```python
from build123d import *

# Parameters (mm, degrees)
SKETCH1_R           = 31.75
SKETCH1_R_2         = 2.05
SKETCH1_R_3         = 1.55
BOSS_EXTRUDE1_DEPTH = 40
SKETCH2_R           = 6.5
CUT_EXTRUDE1_DEPTH  = 30


with BuildPart() as part:
    # Sketch1 → Boss-Extrude1 (new body)
    with BuildSketch(Plane(origin=(0, 0, 0), x_dir=(1, 0, 0), z_dir=(0, 1, 0))):
        with Locations(Location((0, 0, 0), (0, 0, 270))):
            Circle(SKETCH1_R)
        with Locations(Location((0, 0, 0), (0, 0, 270))):
            Circle(SKETCH1_R_2, mode=Mode.SUBTRACT)
        with Locations(Location((0, 12.5, 0), (0, 0, 270))):
            Circle(SKETCH1_R_3, mode=Mode.SUBTRACT)
        with Locations(Location((12.5, 0, 0), (0, 0, 270))):
            Circle(SKETCH1_R_3, mode=Mode.SUBTRACT)
        with Locations(Location((0, -12.5, 0), (0, 0, 270))):
            Circle(SKETCH1_R_3, mode=Mode.SUBTRACT)
        with Locations(Location((-12.5, 0, 0), (0, 0, 270))):
            Circle(SKETCH1_R_3, mode=Mode.SUBTRACT)
        with Locations(Location((19.083044257, 19.083044257, 0), (0, 0, 270))):
            Circle(SKETCH1_R_3, mode=Mode.SUBTRACT)
        with Locations(Location((19.083044257, -19.083044257, 0), (0, 0, 270))):
            Circle(SKETCH1_R_3, mode=Mode.SUBTRACT)
        with Locations(Location((-19.083044257, -19.083044257, 0), (0, 0, 270))):
            Circle(SKETCH1_R_3, mode=Mode.SUBTRACT)
        with Locations(Location((-19.083044257, 19.083044257, 0), (0, 0, 270))):
            Circle(SKETCH1_R_3, mode=Mode.SUBTRACT)
    extrude(amount=BOSS_EXTRUDE1_DEPTH)

    # Sketch2 → Cut-Extrude1 (cut)
    with BuildSketch(Plane.XZ):
        with Locations(Location((0, 0, 0), (0, 0, 270))):
            Circle(SKETCH2_R)
    extrude(amount=-CUT_EXTRUDE1_DEPTH, mode=Mode.SUBTRACT)


solid = part.part
```
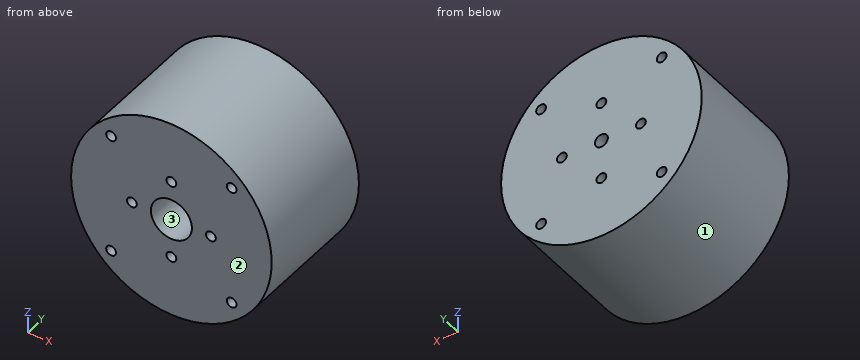
Here's how the part is built. I have some questions about the finished solid (model axes, mm). Face numbers are marked on the shaded views. Give positions to 0.01 mm unless a question says otherwise; leave off trailing zeros. Write each loop counter-clockwise with the first axis right and the second up, starting at its lowest first coordinate (ties: lowest second). Pieces come first, ordered by that corner, then holes.
(1) Imagine slicing it at C-C, the plane y = 7. Count the separate pieces of the cut face and the enclosed holes in it, and give its area (3 significant figures).
Output values:
separate pieces: 1
enclosed holes: 9
area: 2,970 mm2
(2) Imagine slicing it at D-D, the plane x = 12.5. Write out the boundary of the cut face in (y, z).
Output values:
outline: (0, -29.19) - (40, -29.19) - (40, -1.55) - (0, -1.55) - close; (0, 1.55) - (40, 1.55) - (40, 29.19) - (0, 29.19) - close
(3) If I drill on L1, parallel to X at y = 23.75, z = 0; L2, parallel to X at y = 38, z = 20.5; L3, parallel to X at y = 14, z = -12.5, over which ranges is the centre line in solid material (lowest first)?
Output values:
L1: x = -31.75 to -14.05, -10.95 to -6.5, 6.5 to 10.95, 14.05 to 31.75
L2: x = -24.24 to -19.71, -18.45 to 18.45, 19.71 to 24.24
L3: x = -29.19 to -1.55, 1.55 to 29.19
(4) Imagine slicing it at B-B, the plane z = -12.5. Write out the boundary of the cut face in (x, y).
Output values:
outline: (-29.19, 0) - (-1.55, 0) - (-1.55, 40) - (-29.19, 40) - close; (1.55, 0) - (29.19, 0) - (29.19, 40) - (1.55, 40) - close
(5) Will these pins go through, and if not, where does the flat tip stop? pin 1 (3 mm diameter, centred on x = 12.5, y = 8.5, fed in from +Z); pin 2 (5 mm diameter, centred on y = 29, z = -17, fed in from +X); pin 3 (2.5 mm diameter, centred on x = 19.08, z = -19.08, fed in from +Y); pin 4 (4 mm diameter, centred on x = -1.5, z = -2.5, fed in from -Y).
Output values:
pin 1: stops at z = 29.78
pin 2: stops at x = 28.25
pin 3: passes through
pin 4: stops at y = 30
(6) Imagine slicing it at A-A, the plane x = 0. Write out the boundary of the cut face in (y, z), and give its area (3 significant figures).
Output values:
outline: (0, -31.75) - (40, -31.75) - (40, -14.05) - (0, -14.05) - close; (0, -10.95) - (40, -10.95) - (40, -2.05) - (30, -2.05) - (30, -6.5) - (0, -6.5) - close; (0, 6.5) - (30, 6.5) - (30, 2.05) - (40, 2.05) - (40, 10.95) - (0, 10.95) - close; (0, 14.05) - (40, 14.05) - (40, 31.75) - (0, 31.75) - close
area: 1,860 mm2
(7) Thinking about a two-plate mould opening in X: for the marked faces 1, 2 and 3, which applies, pulls with the +X half, pulls with the -X half, needs draft (parallel to the pull), parting line crosses it, or undercut?
Output values:
face 1: parting line crosses it
face 2: needs draft
face 3: undercut
